Drawing for the job (mm, zero at the part's lowest x, y, z). Round coordinates to 2 decimals unless told otherwise and drop trailing zeros. Loops run counter-clockwise (first coordinate to the right, second up) from the corner with the lowest first, then second, coordinate; pieces in that order, holes last. Notation, with made-up numbers: (75, -2.75) -> (121, -2.75) arc R37 ccw to (121, 34.25) -> close; hole circle Ø2 at (26, 86). An arc over 180 degrees is marked (long way). Put each result on its own line as item: value. Start each with the question number.
Item 1: Drill centre lines: probe 1 along Z at (x, y) = (0.25, 6); probe 2 along Y at (x, z) = (0.4, 1.25). Where is each one in solid material? Low to high. Write a range as [from, to].
Item 2: Cut at B-B, the plane y = 6.75. List the corners of the cut face in (x, z), plus the area to 3 significant figures.
Item 3: Cut at A-A, the plane x = 0.2. List the corners of the cut face in (y, z).
Item 4: Cut at C-C, the plane z = 1.3. List the corners of the cut face in (x, y), plus the area to 3 significant figures.
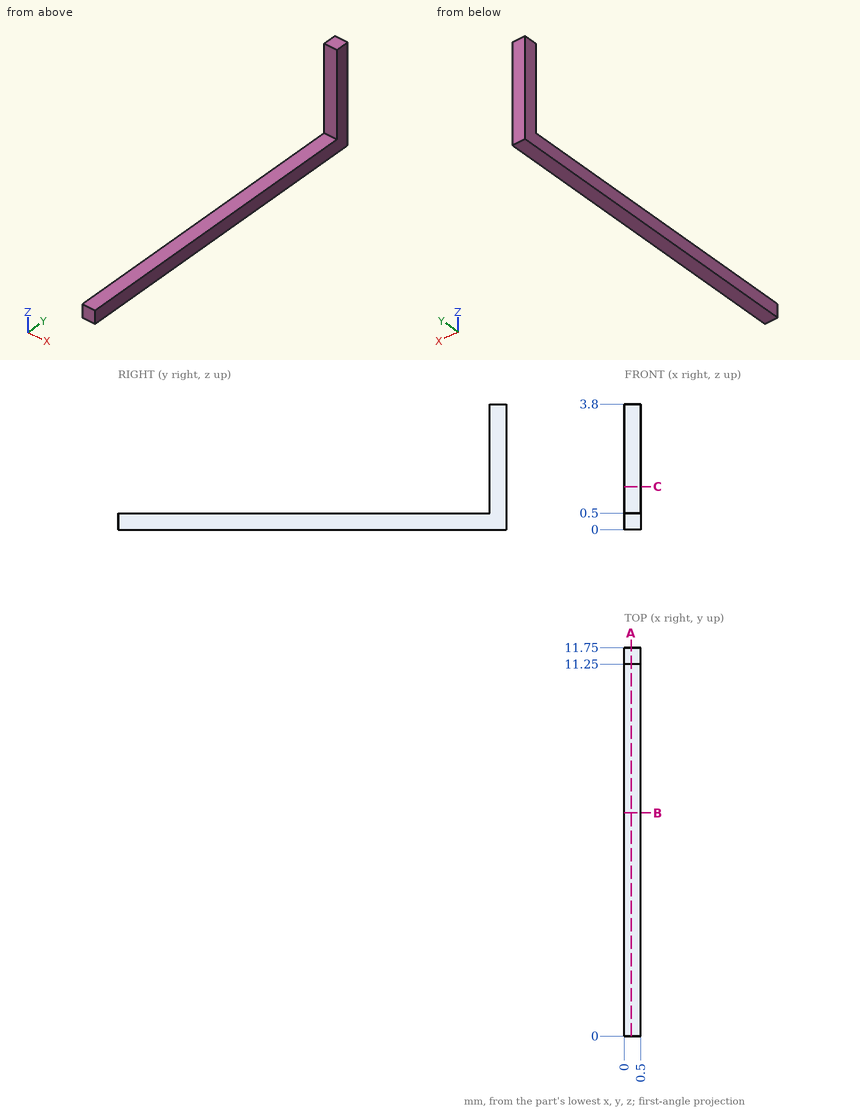
Reply:
1. probe 1: z = [0, 0.5]
1. probe 2: y = [11.25, 11.75]
2. outline: (0, 0) -> (0.5, 0) -> (0.5, 0.5) -> (0, 0.5) -> close
2. area: 0.250 mm^2
3. outline: (0, 0) -> (11.75, 0) -> (11.75, 3.8) -> (11.25, 3.8) -> (11.25, 0.5) -> (0, 0.5) -> close
4. outline: (0, 11.25) -> (0.5, 11.25) -> (0.5, 11.75) -> (0, 11.75) -> close
4. area: 0.250 mm^2
